from build123d import *

# Parameters (mm, degrees)
CYLINDER003_R     = 6
CYLINDER003_DEPTH = 25
CYLINDER002_R     = 6
CYLINDER002_DEPTH = 9
CYLINDER_R        = 6
CYLINDER_DEPTH    = 5


with BuildPart() as cylinder003:
    # Cylinder003 → Cylinder003 (new body)
    with BuildSketch(Plane.XY.offset(9)):
        Circle(CYLINDER003_R)
    extrude(amount=CYLINDER003_DEPTH)


with BuildPart() as cylinder002:
    # Cylinder002 → Cylinder002 (new body)
    with BuildSketch(Plane.XY):
        Circle(CYLINDER002_R)
    extrude(amount=CYLINDER002_DEPTH)


with BuildPart() as fusion:
    # Cylinder → Cylinder (new body)
    with BuildSketch(Plane.XY.offset(-5)):
        Circle(CYLINDER_R)
    extrude(amount=CYLINDER_DEPTH)

    # Fusion: union Cylinder003, Cylinder002
    add(cylinder003.part)
    add(cylinder002.part)


solid = fusion.part
Geometry check sheet. Reference: the model listing, model coordinates, mm. Give positions to 0.01 mm unless a question says otherwise; leave off trailing zeros. Write each loop counter-clockwise with the first axis right and the second up, starting at its lowest first coordinate (ties: lowest second). Pieces come first, ordered by that corner, then holes.
1) Cross-section at C-C (y = 3.5). Record the boundary of the cut face in (x, z).
Values follow:
outline: (-4.87, -5) - (4.87, -5) - (4.87, 34) - (-4.87, 34) - close
2) Cross-section at A-A (z = 5). Record the boundary of the cut face in (x, y), plus the area to 3 significant figures.
Values follow:
outline: circle Ø12 at (0, 0)
area: 113 mm2
3) Go/stop test with flat-tipped pins: pin 1 Ø1 at (x, z) = (2, 24.5) entering from +Y; pin 2 Ø1 at (x, z) = (-1, 2) entering from -Y; pin 3 Ø2 at (y, z) = (1.5, 24.5) entering from +X. Record where each tip stops, or that it passes through.
Values follow:
pin 1: stops at y = 5.81
pin 2: stops at y = -5.98
pin 3: stops at x = 5.98
4) Thickness scan on line 1 (Y direction, x = 3.5, z = -2.5); line 2 (Y direction, x = -2.25, z = 2); line 3 (X direction, y = -3.75, z = 32). Record the ranges inside material, lowest first.
Values follow:
line 1: y = -4.87 to 4.87
line 2: y = -5.56 to 5.56
line 3: x = -4.68 to 4.68
5) Cross-section at B-B (y = -2.75). Record the boundary of the cut face in (x, z), plus the area to 3 significant figures.
Values follow:
outline: (-5.33, -5) - (5.33, -5) - (5.33, 34) - (-5.33, 34) - close
area: 416 mm2
